CAD build for the part. Positions are in the model's coordinates, mm. A direction names the side the tool comes from. Round coordinates to 2 decimals unless told otherwise and drop trailing zeros. Loops run counter-clockwise (first coordinate to the right, second up) from the corner with the lowest first, then second, coordinate; pieces in that order, holes last. Notation, with made-up numbers: M -1.75,28.25 L 9.25,28.25 A20 ccw 9.25,61.25 Z; hole C -21.5,1 d1. An arc over 180 degrees is marked long. Use a Markdown table: item, result. Add a question column.
(1) Flat gauge pins, fed straight in: P1, Ø6.5, axis at x = -75, y = 22, coming from the -Z side; P2, Ø4, axis at x = -25, y = 22.5, coming from the -Z side; P3, Ø5, axis at x = -12.5, y = -6.5, coming from the +Z side. Where does each tip first touch, or does it go through?
(2) Wall check: L1, parallel to Y at x = -73.55, z = 11.9; L2, parallel to X at y = 23.55, z = 6.2; L3, parallel to X at y = 0, z = 2.05. Give the ranges that are in metal, low to high.
(3) Band-saw the part on B-B, the plane x = -50. Write the cut outline in (y, z), and give its area (3 significant figures).
(4) Band-saw the part on A-A, the plane y = -23.55. Write the cut outline in (x, z), and give its area (3 significant figures).
(5) Which spindle directions (+Z, -Z, +X, -X, +Y, -Y) get a long thin tool onto all of the face, cutting with end or side? Do faces 1 (the face through (-14.985, -0.66, 2.465)), 2 (the face through (-69.855, -22.018, 7.958)), 3 (the face through (-13.887, -10.648, 9.93)). Say none if no direction does.
(6) Two-plate mould, pull along X, no slides. Class faces 4 (the face through (-32.403, -7.296, 10.07)), 5 (the face through (-30, -1, 5)), 6 (the face through (80, -1, 7)): released by +X, released by -X, zero draft, split by the parting line, or undercut.
(7) Band-saw the part on D-D, the plane y = 0. Write the cut outline in (x, z).
(8) Band-saw the part on C-C, the plane z = 3. Write the cut outline in (x, y).
from build123d import *

# Parameters (mm, degrees)
F0_W     = 160
F0_H     = 75
F0_R     = 17.5
F1_DEPTH = 15
F2_R     = 2.5
F2_R_2   = 19.05
F3_DEPTH = 25
F4_R     = 4
F5_DEPTH = 11
F6_W     = 60
F6_H     = 5
F7_DEPTH = 79.7
F8_R     = 19
F8_R_2   = 17.5
F8_R_3   = 15
F9_DEPTH = 5


# Not quite as in the source:
# - a feature names something its author has since deleted; it is built from what else it names


with BuildPart() as f1:
    # F0 (on Top) → F1 (new body)
    with BuildSketch(Plane.XY):
        Rectangle(F0_W, F0_H)
        Circle(F0_R, mode=Mode.SUBTRACT)
    extrude(amount=F1_DEPTH)

    # F2 (on face) → F3 (cut)
    with BuildSketch(Plane.XY.offset(15)):
        with Locations((-73.55, 23.55)):
            Circle(F2_R)
        with Locations((-26.45, 23.55)):
            Circle(F2_R)
        with Locations((-26.45, -23.55)):
            Circle(F2_R)
        with Locations((-73.55, -23.55)):
            Circle(F2_R)
        with Locations((-50, 0)):
            Circle(F2_R_2)
    extrude(amount=-F3_DEPTH, mode=Mode.SUBTRACT)

    # F4 (on face) → F5 (cut)
    with BuildSketch(Plane(origin=(0, 0, 0), x_dir=(1, 0, 0), z_dir=(0, 0, -1))):
        with Locations((-73.55, 23.55)):
            Circle(F4_R)
        with Locations((-26.45, 23.55)):
            Circle(F4_R)
        with Locations((-26.45, -23.55)):
            Circle(F4_R)
        with Locations((-73.55, -23.55)):
            Circle(F4_R)
    extrude(amount=-F5_DEPTH, mode=Mode.SUBTRACT)

    # F6 (on face) → F7 (cut)
    with BuildSketch(Plane.XZ.offset(37.5)):
        with Locations((-50, 2.5)):
            Rectangle(F6_W, F6_H)
    extrude(amount=-F7_DEPTH, mode=Mode.SUBTRACT)

    # F8 (on face) → F9 (join)
    with BuildSketch(Plane(origin=(0, 0, 0), x_dir=(1, 0, 0), z_dir=(0, 0, -1))):
        Circle(F8_R)
        Circle(F8_R_2, mode=Mode.SUBTRACT)
        Circle(F8_R_2)
        Circle(F8_R_3, mode=Mode.SUBTRACT)
    extrude(amount=-F9_DEPTH)


solid = f1.part
Return value:
| question | item | result |
|---|---|---|
| 1 | P1 | z = 5 |
| 1 | P2 | z = 11 |
| 1 | P3 | z = 5 |
| 2 | L1 | -37.5 to -26.05, -21.05 to 21.05, 26.05 to 37.5 |
| 2 | L2 | -80 to -77.55, -69.55 to -30.45, -22.45 to 80 |
| 2 | L3 | -20 to -15, 15 to 80 |
| 3 | outline | M -37.5,5 L -19.05,5 L -19.05,15 L -37.5,15 Z; M 19.05,5 L 37.5,5 L 37.5,15 L 19.05,15 Z |
| 3 | area | 369 mm^2 |
| 4 | outline | M -80,5 L -77.55,5 L -77.55,11 L -76.05,11 L -76.05,15 L -80,15 Z; M -71.05,11 L -69.55,11 L -69.55,5 L -30.45,5 L -30.45,11 L -28.95,11 L -28.95,15 L -71.05,15 Z; M -23.95,11 L -22.45,11 L -22.45,5 L -20,5 L -20,0 L 80,0 L 80,15 L -23.95,15 Z |
| 4 | area | 1,960 mm^2 |
| 5 | face 1 | +Z, -Z |
| 5 | face 2 | -Z |
| 5 | face 3 | +Z |
| 6 | face 4 | undercut |
| 6 | face 5 | zero draft |
| 6 | face 6 | released by +X |
| 7 | outline | M -80,5 L -69.05,5 L -69.05,15 L -80,15 Z; M -30.95,5 L -20,5 L -20,0 L -15,0 L -15,5 L -17.5,5 L -17.5,15 L -30.95,15 Z; M 15,0 L 80,0 L 80,15 L 17.5,15 L 17.5,5 L 15,5 Z |
| 8 | outline | M -20,-37.5 L 80,-37.5 L 80,37.5 L -20,37.5 Z; hole C 0,0 d30 |
